Autodesk Fusion 360 part; units mm, degrees
sketch "Sketch1" plane through (0, 0, 0) normal (0, 1, 0) x (1, 0, 0)
  line L0 (0, 0) -> (56, 0)
  line L1 (56, 0) -> (56, -23)
  line L2 (56, -23) -> (0, -23)
  line L3 (0, -23) -> (0, 0)
  dimension "d1" = 56
  dimension "d2" = 23
extrude "Extrude1" add sketch "Sketch1" along normal blind 3
sketch "Sketch2" plane through (0, 3, 0) normal (0, 1, 0) x (-1, 0, 0)
  line L0 (0, 23) -> (-56, 23)
  line L1 (-56, 23) -> (-56, 0)
  line L2 (-56, 0) -> (0, 0)
  line L3 (0, 0) -> (0, 23)
  line L4 (0, 0) -> (-55.9429, 0)
  line L5 (-55.9429, 0) -> (-55.9429, 7.5)
  line L6 (-55.9429, 7.5) -> (0, 7.5)
  line L7 (0, 7.5) -> (0, 0)
  line L8 (0, 11.5) -> (-56, 11.5)
  line L9 (-55.9429, 15.5) -> (0, 15.5)
  line L10 (0, 15.5) -> (0, 23)
  line L11 (0, 23) -> (-56, 23)
  line L12 (-55.9429, 15.5) -> (-56, 23)
  line L13 (0, 7.5) -> (-7.5, 7.5)
  line L14 (-7.5, 7.5) -> (-7.5, 4.5)
  line L15 (-55.9429, 7.5) -> (-48.4429, 7.5)
  line L16 (-48.4429, 7.5) -> (-48.4429, 4.5)
  line L17 (-7.5, 4.5) -> (-48.4429, 4.5)
  line L18 (-48.4429, 4.5) -> (-48.4429, 7.5)
  line L19 (-7.5, 18.5) -> (-48.4429, 18.5)
  line L20 (-48.4429, 15.5) -> (-48.4429, 18.5)
  line L21 (-7.5, 15.5) -> (-7.5, 18.5)
  line L22 (0, 0) -> (0, 3)
  line L23 (0, 3) -> (-56, 3)
  line L24 (0, 20) -> (-56, 20)
  dimension "d5" = 7.5
  dimension "d6" = 7.5
  dimension "d7" = 3
  dimension "d8" = 7.5
  dimension "d9" = 3
  dimension "d10" = 3
extrude "Extrude2" add sketch "Sketch2" along normal blind 6.5 contours L0 L3 L10 L11 L12 L24 | L2 L3 L4 L5 L7 L22 L23
sketch "Sketch3" plane through (0, 0, 0) normal (0, 0, -1) x (-1, 0, 0)
  line L0 (-56, 0) -> (0, 0)
  line L1 (0, 0) -> (0, 9.5)
  line L2 (0, 9.5) -> (-55.9429, 9.5)
  line L3 (-55.9429, 9.5) -> (-55.9429, 3)
  line L4 (-55.9429, 3) -> (-56, 3)
  line L5 (-56, 3) -> (-56, 0)
  line L6 (0, 0) -> (0, 9.5)
  line L7 (0, 9.5) -> (-7, 9.5)
  line L8 (-7, 9.5) -> (-7, 6.5)
  line L9 (-55.9429, 9.5) -> (-48.9429, 9.5)
  line L10 (-48.9429, 9.5) -> (-48.9429, 6.5)
  line L11 (-7, 6.5) -> (-48.9429, 6.5)
  dimension "d13" = 9.5
  dimension "d14" = 7
  dimension "d15" = 3
  dimension "d16" = 7
  dimension "d17" = 3
extrude "Extrude3" cut sketch "Sketch3" against normal blind 30 contours L2 L8 L10 L11
sketch "Sketch4" plane through (0, 0, 0) normal (0, 0, -1) x (-1, 0, 0)
  line L0 (-7, 9.5) -> (-7, 6.5)
  line L1 (-7, 6.5) -> (-48.9429, 6.5)
  line L2 (-48.9429, 6.5) -> (-48.9429, 9.5)
  line L3 (-48.9429, 9.5) -> (-55.9429, 9.5)
  line L4 (-55.9429, 9.5) -> (-55.9429, 3)
  line L5 (-55.9429, 3) -> (-56, 3)
  line L6 (-56, 3) -> (-56, 0)
  line L7 (-56, 0) -> (0, 0)
  line L8 (0, 0) -> (0, 9.5)
  line L9 (0, 9.5) -> (-7, 9.5)
  line L10 (0, 0) -> (-3.081, 0)
  line L11 (-3.081, 0) -> (-3.081, 9.5)
  line L12 (0, 0) -> (0, 2.916)
  line L13 (0, 2.916) -> (-5.2666, 2.916)
  line L14 (-28, 0) -> (-27.9715, 6.5)
  line L15 (-2.393, 9.5) -> (-2.393, 6.584)
  line L16 (-2.393, 6.584) -> (-5.7836, 6.584)
  line L17 (-3.081, 0) -> (-3.081, 4.5)
  line L18 (-3.081, 0) -> (-3.081, 5.5)
  circle A0 centre (-3.081, 5.5) radius 1.5
  circle A1 centre (-52.8697, 5.7187) radius 1.5
  dimension "d20" = 3.081
  dimension "d21" = 2.916
  dimension "d23" = 2.916
  dimension "d25" = 4.5
  dimension "d26" = 5.5
  dimension "d27" = 3
extrude "Extrude4" cut sketch "Sketch4" against normal blind 30 contours L11 L15 L16 A0 | L11 L16 A0 | L11 L15 L16 L17 L18 A0 | L11 L16 L17 L18 A0 | A1
sketch "Sketch6" plane through (0, 3, 0) normal (0, 1, 0) x (-1, 0, 0)
  line L0 (-55.9772, 20) -> (-56, 23)
  line L1 (-56, 23) -> (-56, 0)
  line L2 (-56, 0) -> (-55.9429, 0)
  line L3 (-55.9429, 0) -> (-55.9429, 3)
  line L4 (-55.9429, 3) -> (0, 3)
  line L5 (0, 3) -> (0, 20)
  line L6 (0, 20) -> (-55.9772, 20)
  line L7 (-55.9772, 20) -> (-47.9772, 20)
  line L8 (-47.9772, 20) -> (-37.9772, 20)
  line L9 (-37.9772, 20) -> (-37.9772, 10)
  line L10 (-37.9772, 10) -> (-47.9772, 10)
  line L11 (-47.9772, 10) -> (-47.9772, 20)
  line L12 (-37.9772, 20) -> (-37.9772, 19.4199)
  line L13 (-37.9772, 3) -> (-37.9772, 20)
  line L14 (-37.9772, 20) -> (-37.9772, 11.5)
  line L15 (-37.9772, 17) -> (-37.9772, 8.5)
  line L16 (-37.9772, 17) -> (-37.9772, 7)
  line L17 (-37.9772, 7) -> (-47.9772, 7)
  line L18 (-47.9772, 7) -> (-47.9772, 17)
  line L19 (-47.9772, 17) -> (-37.9772, 17)
  dimension "d30" = 8
  dimension "d31" = 10
  dimension "d32" = 10
  dimension "d38" = 10
  dimension "d39" = 10
extrude "Extrude5" add sketch "Sketch6" along normal blind 7.5 contours L9 L10 L11 L13 L14 L15 L16 L18 L19 | L10 L13 L15 L16 L17 L18
sketch "Sketch7" plane through (47.9772, 0, 0) normal (1, 0, 0) x (0, 0, -1)
  line L0 (-17, 3) -> (-7, 3)
  line L1 (-7, 10.5) -> (-17, 10.5)
  circle A0 centre (-12, 10.5) radius 3
  line L2 (-7, 3) -> (-7, 10.5)
  line L3 (-17, 10.5) -> (-17, 3)
  dimension "d35" = 6
extrude "Extrude6" cut sketch "Sketch7" against normal blind 10 contours L1 A0 picked at (-12.5, 9.634)
Check sheet for the modelled part. Datum: model origin and axes. Units: mm. A direction names the side the tool comes from. Coordinates: 2 decimals unless noted, no trailing zeros. Write each loop counter-clockwise with the first axis right and the second up, starting at its lowest first coordinate (ties: lowest second). Pieces come first, ordered by that corner, then holes. Notation, with made-up numbers: (-39.5, 77) -> (0.5, 77) arc R21 ccw to (0.5, 112) -> close; hole circle Ø10 at (35.25, 86). An arc over 180 degrees is marked (long way). Use a Markdown table: item, result.
1. Sectioned sample at C-C (y = 8). Enter the section's corners in (x, z).
Reported:
| item | result |
|---|---|
| outline | (0, 0) -> (7, 0) -> (7, 3) -> (0, 3) -> close; (0, 20) -> (7, 20) -> (7, 23) -> (0, 23) -> close; (37.98, 7) -> (47.98, 7) -> (47.98, 10.34) -> (37.98, 10.34) -> close; (37.98, 13.66) -> (47.98, 13.66) -> (47.98, 17) -> (37.98, 17) -> close; (48.94, 0) -> (55.94, 0) -> (55.94, 3) -> (48.94, 3) -> close; (48.94, 20) -> (55.98, 20) -> (56, 23) -> (48.94, 23) -> close |
2. Sectioned sample at A-A (z = 12). Enter the section's corners in (x, y), plus the area to 3 significant figures.
Reported:
| item | result |
|---|---|
| outline | (0, 0) -> (56, 0) -> (56, 3) -> (47.98, 3) -> (47.98, 7.5) -> (37.98, 7.5) -> (37.98, 3) -> (0, 3) -> close |
| area | 213 mm2 |
3. Sectioned sample at D-D (z = 21.75). Give the number of separate pieces and of enclosed holes in the cut face, plus the area to 3 significant figures.
Reported:
| item | result |
|---|---|
| separate pieces | 1 |
| enclosed holes | 2 |
| area | 392 mm2 |
4. Sectioned sample at B-B (x = 43.5). Enter the section's corners in (y, z).
Reported:
| item | result |
|---|---|
| outline | (0, 0) -> (6.5, 0) -> (6.5, 3) -> (3, 3) -> (3, 7) -> (10.5, 7) -> (10.5, 9) arc R3 cw to (10.5, 15) -> (10.5, 17) -> (3, 17) -> (3, 20) -> (6.5, 20) -> (6.5, 23) -> (0, 23) -> close |
5. Go/stop test with flat-tipped pins: pin 1 Ø1.5 at (x, z) = (51.5, 2) entering from +Y; pin 2 Ø3 at (x, z) = (23.5, 14) entering from +Y; pin 3 Ø2.5 at (x, z) = (25.5, 21.5) entering from +Y. Record where each tip stops, or that it passes through.
Reported:
| item | result |
|---|---|
| pin 1 | stops at y = 9.5 |
| pin 2 | stops at y = 3 |
| pin 3 | stops at y = 6.5 |
6. Tool access check on faces 1 (the flat face through (7, 8, 21)), 2 (the flat face through (43, 10.5, 16)), 3 (the flat face through (47.977, 6, 12)), 4 (the flat face through (28, 6.5, 1)), 5 (the flat face through (43, 7, 17)). Record the directions out of +Z, -Z, +X, -X, +Y, -Y that give a thin tool (end or side, any length) a straight path to the whole face; none if there is none.
Reported:
| item | result |
|---|---|
| face 1 | +Z, -Z, +Y |
| face 2 | +Z, -Z, +X, -X, +Y |
| face 3 | +X, +Y |
| face 4 | -Z, +Y |
| face 5 | +X, -X, +Y |
7. Scan lines: line 1 along Z through (x, y) = (36, 4.75); line 2 along X through (y, z) = (8.25, 20.5); line 3 along X through (y, z) = (5.5, 1.05). Record each from-to range of solid material in increasing order.
Reported:
| item | result |
|---|---|
| line 1 | z = 0 to 3, 20 to 23 |
| line 2 | x = 0 to 7, 48.94 to 55.98 |
| line 3 | x = 0 to 1.58, 4.58 to 51.39, 54.35 to 55.94 |
8. Release check for a two-part mould opening along Z. For faces 6 (the flat face through (28, 4, 23)), 7 (the flat face through (43, 10.5, 8)), 8 (the flat face through (28, 5, 3)) record: pulls with the +Z half, pulls with the -Z half, needs draft (parallel to the pull), parting line crosses it, or undercut.
Reported:
| item | result |
|---|---|
| face 6 | pulls with the +Z half |
| face 7 | needs draft |
| face 8 | undercut |
